Geometry check sheet. Reference: the model listing, model coordinates, mm. Face numbers are marked on the shaded views. A direction names the side the tool comes from. Coordinates: 2 decimals unless noted, no trailing zeros. Loops run counter-clockwise (first coordinate to the right, second up) from the corner with the lowest first, then second, coordinate; pieces in that order, holes last. Notation, with made-up numbers: M -26.75,72 L -13.75,72 A14 ccw -13.75,99 Z; hole C 36,66 d6. An arc over 180 degrees is marked long. One line per question, with ' | ' between items. Start each with the question number.
from build123d import *

# Parameters (mm, degrees)
F1_DEPTH = 100
F2_DEPTH = 100
F3_DEPTH = 100


with BuildPart() as f1:
    # F0 (on Front) → F1 (new body)
    with BuildSketch(Plane.XZ):
        Polygon((-177.0265877346, -438.935896764), (1280.8620243115, -438.935896764), (1322.9734122654, -338.935896764), (-177.0265877346, -338.935896764), align=None)
    extrude(amount=F1_DEPTH)

    # F0 (on Front) → F2 (join)
    with BuildSketch(Plane.XZ):
        Polygon((-177.0265877346, -338.935896764), (-345.4721395502, -738.935896764), (-303.3607515963, -738.935896764), (-177.0265877346, -438.935896764), align=None)
        Polygon((-345.4721395502, -738.935896764), (-429.694915458, -938.935896764), (-387.5835275041, -938.935896764), (-303.3607515963, -738.935896764), align=None)
        Polygon((-429.694915458, -938.935896764), (-429.694915458, -1038.935896764), (-387.5835275041, -938.935896764), align=None)
    extrude(amount=F2_DEPTH)

    # F0 (on Front) → F3 (join)
    with BuildSketch(Plane.XZ):
        Polygon((1280.8620243115, -438.935896764), (1322.9734122654, -438.935896764), (1322.9734122654, -338.935896764), align=None)
        Polygon((1070.305084542, -938.935896764), (1070.305084542, -1038.935896764), (1322.9734122654, -438.935896764), (1280.8620243115, -438.935896764), (1154.5278604498, -738.935896764), align=None)
        Polygon((-387.5835275041, -938.935896764), (-429.694915458, -1038.935896764), (1070.305084542, -1038.935896764), (1070.305084542, -938.935896764), align=None)
    extrude(amount=F3_DEPTH)


solid = f1.part
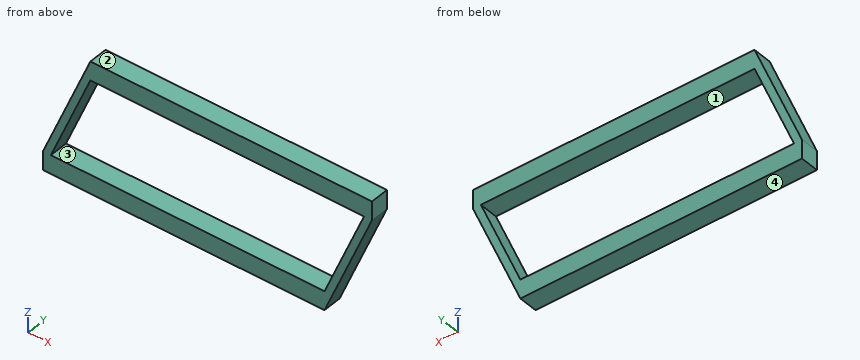
1. Thickness scan on line 1 (Z direction, x = 221, y = -59); line 2 (X direction, y = -61, z = -533); line 3 (X direction, y = -82, z = -645.5). Record the ranges inside material, lowest first.
2. Sectioned sample at C-C (z = -740). Record the cut outline in (x, y), and give its area (3 significant figures).
3. Tool access check on the marked faces 1 and 2. Record the directions out of +Z, -Z, +X, -X, +Y, -Y that give a thin tool (end or side, any length) a straight path to the whole face; none if there is none.
4. Sectioned sample at A-A (x = 128). Record the cut outline in (y, z).
5. Depth check by flat-ended pin: pin 1 Ø5 at (y, z) = (-60, -551) entering from +X; pin 2 Ø10 at (y, z) = (-30, -865) entering from -X; pin 3 Ø3 at (x, z) = (622, -954) entering from +Y. Enter the tip coordinate at first touch or a pass-through.
6. Draft check along X on the marked faces 3 and 4. Enter one of: +X half, -X half, draft (parallel to the pull), parting line (faces both ways), or undercut.
7. Sectioned sample at B-B (y = -17). Record the cut outline in (x, z), and give its area (3 significant figures).
Result:
1) line 1: z = -1038.94 to -938.94, -438.94 to -338.94 | line 2: x = -258.75 to -216.64, 1241.25 to 1283.36 | line 3: x = -306.12 to -264.01, 1193.88 to 1235.99
2) outline: M -345.92,-100 L -303.81,-100 L -303.81,0 L -345.92,0 Z; M 1154.08,-100 L 1196.19,-100 L 1196.19,0 L 1154.08,0 Z | area: 8,420 mm2
3) face 1: +Y, -Y | face 2: +Z, +X, -X, +Y, -Y
4) outline: M -100,-1038.94 L 0,-1038.94 L 0,-938.94 L -100,-938.94 Z; M -100,-438.94 L 0,-438.94 L 0,-338.94 L -100,-338.94 Z
5) pin 1: stops at x = 1276.83 | pin 2: stops at x = -400.67 | pin 3: stops at y = 0
6) face 3: undercut | face 4: draft
7) outline: M -429.69,-1038.94 L 1070.31,-1038.94 L 1322.97,-438.94 L 1322.97,-338.94 L -177.03,-338.94 L -429.69,-938.94 Z; hole M -387.58,-938.94 L 1070.31,-938.94 L 1280.86,-438.94 L -177.03,-438.94 Z | area: 346,000 mm2
